Model file for the job. Use its own axes, mm. A direction names the side the tool comes from. Round coordinates to 2 decimals unless told otherwise and drop trailing zeros. Loops run counter-clockwise (first coordinate to the right, second up) from the corner with the lowest first, then second, coordinate; pieces in that order, holes last.
from build123d import *

# Parameters (mm, degrees)
SKETCH1_W                                     = 177.8
SKETCH1_H                                     = 177.8
BOSS_EXTRUDE1_DEPTH                           = 12.7
F_13_32_0_40625_DIAMETER_HOLE1_D              = 10.31875
F_13_32_0_40625_DIAMETER_HOLE1_DEPTH          = 25.4
F_13_32_0_40625_DIAMETER_HOLE1_TIP            = 3.100065256
SKETCH4_R                                     = 58.7375
CUT_EXTRUDE1_DEPTH                            = 127.363404513
SKETCH5_OUTSIDE_W                             = 230.154
SKETCH5_OUTSIDE_H                             = 230.154
SKETCH5_OUTSIDE_R                             = 88.9
CUT_EXTRUDE2_DEPTH                            = 12.7
CBORE_FOR_1_4_SOCKET_HEAD_CAP_SCREW1_AT_COUNT = 2
CBORE_FOR_1_4_SOCKET_HEAD_CAP_SCREW1_AT_PITCH = 101.6
CBORE_FOR_1_4_SOCKET_HEAD_CAP_SCREW1_2_COUNT  = 2
CBORE_FOR_1_4_SOCKET_HEAD_CAP_SCREW1_2_PITCH  = 101.6
CBORE_FOR_1_4_SOCKET_HEAD_CAP_SCREW1_3_COUNT  = 2
CBORE_FOR_1_4_SOCKET_HEAD_CAP_SCREW1_3_PITCH  = 143.684097937


with BuildPart() as part:
    # Sketch1 → Boss-Extrude1 (new body)
    with BuildSketch(Plane(origin=(0, 0, 0), x_dir=(1, 0, 0), z_dir=(0, 1, 0))):
        Rectangle(SKETCH1_W, SKETCH1_H)
    extrude(amount=BOSS_EXTRUDE1_DEPTH)

    # 13/32 (0.40625) Diameter Hole1
    with Locations(Plane(origin=(-52.759004711, 12.7, -52.759004711), x_dir=(0, 0, 1), z_dir=(0, 1, 0))):
        with Locations((0, 0), (0, 105.518009422), (105.518009422, 105.518009422), (105.518009422, 0)):
            Hole(F_13_32_0_40625_DIAMETER_HOLE1_D / 2, depth=F_13_32_0_40625_DIAMETER_HOLE1_DEPTH)
            with Locations((0, 0, -(F_13_32_0_40625_DIAMETER_HOLE1_DEPTH + F_13_32_0_40625_DIAMETER_HOLE1_TIP / 2))):  # 118° drill point
                Cone(0, F_13_32_0_40625_DIAMETER_HOLE1_D / 2, F_13_32_0_40625_DIAMETER_HOLE1_TIP, mode=Mode.SUBTRACT)

    # Sketch4 → Cut-Extrude1 (cut, through all)
    with BuildSketch(Plane(origin=(0, 12.7, 0), x_dir=(1, 0, 0), z_dir=(0, 1, 0))):
        with Locations(Location((0, 0, 0), (0, 0, 270))):
            Circle(SKETCH4_R)
    extrude(amount=-CUT_EXTRUDE1_DEPTH, mode=Mode.SUBTRACT)

    # Sketch5 outside → Cut-Extrude2 (cut)
    with BuildSketch(Plane(origin=(0, 12.7, 0), x_dir=(1, 0, 0), z_dir=(0, 1, 0))):
        Rectangle(SKETCH5_OUTSIDE_W, SKETCH5_OUTSIDE_H)
        with Locations(Location((0, 0, 0), (0, 0, 270))):
            Circle(SKETCH5_OUTSIDE_R, mode=Mode.SUBTRACT)
    extrude(amount=-CUT_EXTRUDE2_DEPTH, mode=Mode.SUBTRACT)

    # Sketch9 → CBORE for 1/4 Socket Head Cap Screw1 (revolve, cut)
    with BuildSketch(Plane(origin=(0, 12.7, -71.842048969), x_dir=(0, 0, 1), z_dir=(1, 0, 0))):
        Polygon((0, 0), (0, 12.7), (3.3782, 12.7), (3.3782, 6.35), (5.55625, 6.35), (5.55625, 0.635), (6.19125, 0), align=None)
    cbore_for_1_4_socket_head_cap_screw1 = revolve(axis=Axis((0, 19.05, -71.842048969), (0, -1, 0)), mode=Mode.SUBTRACT)

    # CBORE for 1/4 Socket Head Cap Screw1 at: CBORE for 1/4 Socket Head Cap Screw1 ×2
    with Locations(*[Vector(0.7071067811865476, 0, 0.7071067811865476) * (i * CBORE_FOR_1_4_SOCKET_HEAD_CAP_SCREW1_AT_PITCH) for i in range(1, CBORE_FOR_1_4_SOCKET_HEAD_CAP_SCREW1_AT_COUNT)]):
        add(cbore_for_1_4_socket_head_cap_screw1, mode=Mode.SUBTRACT)

    # CBORE for 1_4 Socket Head Cap Screw1 2: CBORE for 1/4 Socket Head Cap Screw1 ×2
    with Locations(*[Vector(-0.7071067811865475, 0, 0.7071067811865476) * (i * CBORE_FOR_1_4_SOCKET_HEAD_CAP_SCREW1_2_PITCH) for i in range(1, CBORE_FOR_1_4_SOCKET_HEAD_CAP_SCREW1_2_COUNT)]):
        add(cbore_for_1_4_socket_head_cap_screw1, mode=Mode.SUBTRACT)

    # CBORE for 1_4 Socket Head Cap Screw1 3: CBORE for 1/4 Socket Head Cap Screw1 ×2
    with Locations(*[(0, 0, i * CBORE_FOR_1_4_SOCKET_HEAD_CAP_SCREW1_3_PITCH) for i in range(1, CBORE_FOR_1_4_SOCKET_HEAD_CAP_SCREW1_3_COUNT)]):
        add(cbore_for_1_4_socket_head_cap_screw1, mode=Mode.SUBTRACT)


solid = part.part
Q1. Pull direction X, two halves, no side cores. Call faces 3 (the face through (-68, 6.35, 0)), 4 (the face through (74.96, 6.44, 47.79)): pulls with the +X half, pulls with the -X half, needs draft (parallel to the pull), parting line crosses it, or undercut.
Q2. Slice it at A-A on x = 0. State how many separate pieces and enclosed holes the cut face has, plus the area to 3 significant figures.
Q3. Flat gauge pins, fed straight in: P1, Ø5.5, axis at x = 70, z = -0.5, coming from the +Y side; P2, Ø1.5, axis at x = -18, z = 66, coming from the -Y side; P3, Ø6, axis at x = 59, y = 4, coming from the +Z side (3 decimals); P4, Ø1, axis at y = 4.5, z = -43.5, coming from the +X side. Where does each tip first touch, or does it go through?
Q4. Tool access for faces 1 (the face through (57.874, 6.261, -52.087)), 2 (the face through (4, 6.35, 72)): list every direction of +Z, -Z, +X, -X, +Y, -Y with a clear straight run to the whole face (end or side of a thin tool).
Q5. Slice it at D-D on x = 36.5. Give the cut face in (y, z), plus the area to 3 significant figures.
Q6. Probe line 1 (Z direction, x = -0.5, y = 5.75); line 2 (X direction, y = 4.5, z = 0); line 3 (Z direction, x = -49, y = 5.5). List the from-to ranges inside material, lowest first.
Reply:
1. face 3: undercut
1. face 4: parting line crosses it
2. separate pieces: 4
2. enclosed holes: 0
2. area: 538 mm2
3. P1: stops at y = 6.35
3. P2: stops at y = 0
3. P3: stops at z = 69.045
3. P4: stops at x = 77.81
4. face 1: +Y, -Y
4. face 2: +Y
5. outline: (0, -81.06) - (12.7, -81.06) - (12.7, -46.02) - (0, -46.02) - close; (0, 46.02) - (12.7, 46.02) - (12.7, 81.06) - (0, 81.06) - close
5. area: 890 mm2
6. line 1: z = -88.9 to -75.18, -68.5 to -58.74, 58.74 to 68.5, 75.18 to 88.9
6. line 2: x = -88.9 to -75.22, -68.46 to -58.74, 58.74 to 68.46, 75.22 to 88.9
6. line 3: z = -74.18 to -56.29, -49.23 to -32.39, 32.39 to 49.23, 56.29 to 74.18
